Check sheet for the drawn part. Datum: minimum x, y, z corner. Units: mm. Coordinates: 2 decimals unless noted, no trailing zeros. Loops run counter-clockwise (first coordinate to the right, second up) from the corner with the lowest first, then second, coordinate; pieces in that order, holes last. Notation, with made-up numbers: M -36.5,67.5 L 10.5,67.5 A29 ccw 10.5,98.5 Z; hole C 42.5,67 d6. An arc over 180 degrees is marked long. Answer in a Markdown table with one row per item. Add a question column.
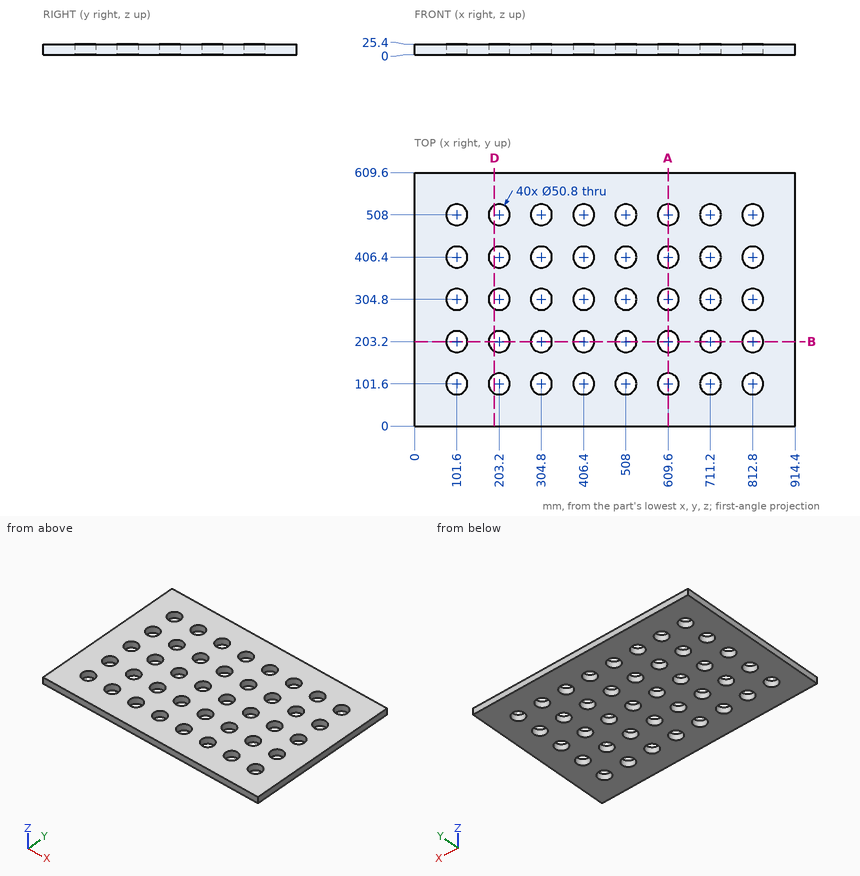
Q1. Cross-section at B-B (y = 203.2). Count the separate pieces of the cut face and the enclosed holes in it, plus the area to 3 significant figures.
Q2. Cross-section at D-D (x = 192). Record the cut outline in (y, z), plus the area to 3 significant figures.
Q3. Cross-section at A-A (x = 609.6). Record the cut outline in (y, z), plus the area to 3 significant figures.
Q4. Thickness scan on L1, parallel to Y at x = 407, z = 23.25; L2, parallel to Y at x = 607, z = 22.75. Record the ranges inside material, lowest first.
Q5. Go/stop test with a flat-tipped pin: pin 1 (8 mm diameter, centred on y = 222.5, z = 4, fed in from -X). Record where the tip stops, or that it passes through.
Answer key:
| question | item | result |
|---|---|---|
| 1 | separate pieces | 9 |
| 1 | enclosed holes | 0 |
| 1 | area | 12,900 mm^2 |
| 2 | outline | M 0,0 L 78.8,0 L 78.8,25.4 L 0,25.4 Z; M 124.4,0 L 180.4,0 L 180.4,25.4 L 124.4,25.4 Z; M 226,0 L 282,0 L 282,25.4 L 226,25.4 Z; M 327.6,0 L 383.6,0 L 383.6,25.4 L 327.6,25.4 Z; M 429.2,0 L 485.2,0 L 485.2,25.4 L 429.2,25.4 Z; M 530.8,0 L 609.6,0 L 609.6,25.4 L 530.8,25.4 Z |
| 2 | area | 9,690 mm^2 |
| 3 | outline | M 0,0 L 76.2,0 L 76.2,25.4 L 0,25.4 Z; M 127,0 L 177.8,0 L 177.8,25.4 L 127,25.4 Z; M 228.6,0 L 279.4,0 L 279.4,25.4 L 228.6,25.4 Z; M 330.2,0 L 381,0 L 381,25.4 L 330.2,25.4 Z; M 431.8,0 L 482.6,0 L 482.6,25.4 L 431.8,25.4 Z; M 533.4,0 L 609.6,0 L 609.6,25.4 L 533.4,25.4 Z |
| 3 | area | 9,030 mm^2 |
| 4 | L1 | 0 to 76.21, 126.99 to 177.81, 228.59 to 279.41, 330.19 to 381.01, 431.79 to 482.61, 533.39 to 609.6 |
| 4 | L2 | 0 to 76.33, 126.87 to 177.93, 228.47 to 279.53, 330.07 to 381.13, 431.67 to 482.73, 533.27 to 609.6 |
| 5 | pin 1 | x = 0 |
